Check sheet for the drawn part. Datum: minimum x, y, z corner. Units: mm. A direction names the side the tool comes from. Give positions to 0.01 mm unless a question says otherwise; leave off trailing zeros. Write each loop counter-clockwise with the first axis right and the second up, starting at its lowest first coordinate (ties: lowest second). Pieces come first, ordered by that corner, then holes. Notation, with made-up numbers: (48, -20) - (55, -20) arc R28 ccw to (55, -1) - close; hole circle Ø10 at (63, 69.25). An arc over 180 degrees is marked (long way). Answer as a JSON object with one key per item and string values. Group by question number.
Item 1: Sectioned sample at A-A, the plane x = 40. Record the boundary of the cut face in (y, z), and give its area (4 significant figures).
Item 2: Scan lines: line 1 along Z through (x, y) = (40, 97); line 2 along X through (y, z) = (72, 39); line 3 along Y through (x, z) = (51, 6). Record each from-to range of solid material in increasing order. Write a range as [from, to].
Item 3: Go/stop test with flat-tipped pins: pin 1 (8 mm diameter, centred on x = 19.5, y = 95.5, fed in from +Z); pin 2 (1 mm diameter, centred on x = 33.5, y = 56, fed in from +Z); pin 3 (12 mm diameter, centred on x = 54.5, y = 110.5, fed in from -Z). Record where each tip stops, or that it passes through.
Item 4: Tool access check on the marked faces 1 and 2. Record the directions out of +Z, -Z, +X, -X, +Y, -Y that give a thin tool (end or side, any length) a straight path to the whole face; none if there is none.
Item 5: Sectioned sample at B-B, the plane z = 40. Record the boundary of the cut face in (x, y).
Item 6: Sectioned sample at D-D, the plane x = 9.5. Record the boundary of the cut face in (y, z), and give its area (3 significant figures).
Item 7: Sectioned sample at C-C, the plane y = 30. Record the boundary of the cut face in (x, z).
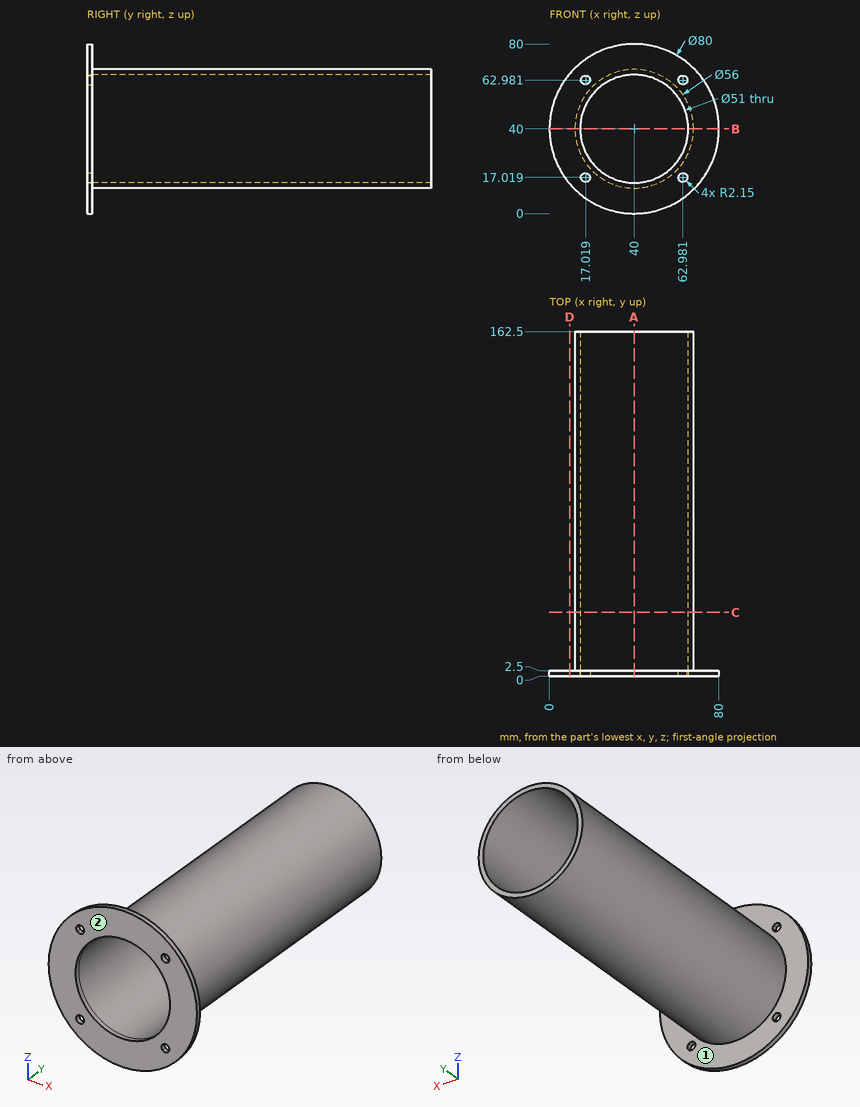
Geometry check:
{
 "1": {"outline": "(0, 0) - (2.5, 0) - (2.5, 12) - (162.5, 12) - (162.5, 14.5) - (0, 14.5) - close; (0, 65.5) - (162.5, 65.5) - (162.5, 68) - (2.5, 68) - (2.5, 80) - (0, 80) - close", "area": "872.5 mm^2"},
 "2": {"line 1": "[12, 14.5], [65.5, 68]", "line 2": "[12.02, 14.52], [65.48, 67.98]", "line 3": "[0, 2.5]"},
 "3": {"pin 1": "z = 62.62", "pin 2": "z = 67.35", "pin 3": "z = 13.32"},
 "4": {"face 1": "+Y", "face 2": "+Z, -Z, +X, -X, -Y"},
 "5": {"outline": "(0, 0) - (14.5, 0) - (14.5, 162.5) - (12, 162.5) - (12, 2.5) - (0, 2.5) - close; (65.5, 0) - (80, 0) - (80, 2.5) - (68, 2.5) - (68, 162.5) - (65.5, 162.5) - close"},
 "6": {"outline": "(0, 14.12) - (2.5, 14.12) - (2.5, 65.88) - (0, 65.88) - close", "area": "129 mm^2"},
 "7": {"outline": "circle Ø56 at (40, 40); hole circle Ø51 at (40, 40)"}
}
